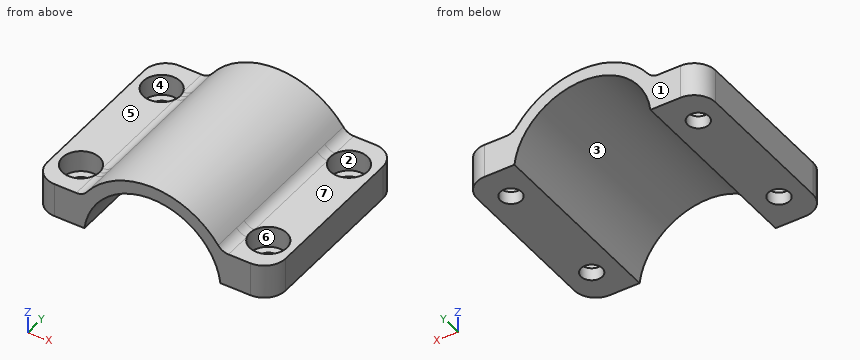
```python
from build123d import *

# Parameters (mm, degrees)
F1_DEPTH = 45
F2_R     = 2.5
F2_R_2   = 4.35
F3_DEPTH = 5
F4_DEPTH = 8.001
F5_R     = 3
F6_R     = 5


with BuildPart() as f1:
    # F0 (on Front) → F1 (new body)
    with BuildSketch(Plane.XZ):
        with BuildLine():
            Line((-28, 10), (-28, 2))
            Line((-28, 2), (-15.975293, 2))
            ThreePointArc((-15.975293, 2), (0, 16.1), (15.975293, 2))
            Line((15.975293, 2), (28, 2))
            Line((28, 2), (28, 10))
            Line((28, 10), (16.272984, 10))
            ThreePointArc((16.272984, 10), (0, 19.1), (-16.272984, 10))
            Line((-16.272984, 10), (-28, 10))
        make_face()
    extrude(amount=F1_DEPTH)

    # F2 (on face) → F3 (cut)
    with BuildSketch(Plane.XY.offset(10)):
        with Locations((-22, -8)):
            Circle(F2_R)
        with Locations((-22, -8)):
            Circle(F2_R_2)
        with Locations((-22, -8)):
            Circle(F2_R, mode=Mode.SUBTRACT)
        with Locations((22, -8)):
            Circle(F2_R)
        with Locations((22, -8)):
            Circle(F2_R_2)
        with Locations((22, -8)):
            Circle(F2_R, mode=Mode.SUBTRACT)
        with Locations((22, -37)):
            Circle(F2_R)
        with Locations((22, -37)):
            Circle(F2_R_2)
        with Locations((22, -37)):
            Circle(F2_R, mode=Mode.SUBTRACT)
        with Locations((-22, -37)):
            Circle(F2_R)
        with Locations((-22, -37)):
            Circle(F2_R_2)
        with Locations((-22, -37)):
            Circle(F2_R, mode=Mode.SUBTRACT)
    extrude(amount=-F3_DEPTH, mode=Mode.SUBTRACT)

    # F2 (on face) → F4 (cut, through all)
    with BuildSketch(Plane.XY.offset(10)):
        with Locations((-22, -8)):
            Circle(F2_R)
        with Locations((22, -8)):
            Circle(F2_R)
        with Locations((-22, -37)):
            Circle(F2_R)
        with Locations((22, -37)):
            Circle(F2_R)
    extrude(amount=-F4_DEPTH, mode=Mode.SUBTRACT)

    # F5
    f5_edges = [f1.edges().sort_by_distance(p)[0] for p in [
        (-16.272984, -22.5, 10),
        (16.272984, -22.5, 10),
    ]]
    fillet(f5_edges, radius=F5_R)

    # F6
    f6_edges = [f1.edges().sort_by_distance(p)[0] for p in [
        (28, -45, 6),
        (28, 0, 6),
        (-28, -45, 6),
        (-28, 0, 6),
    ]]
    fillet(f6_edges, radius=F6_R)


solid = f1.part
```
Geometry: final body of the model. Coordinates: model frame, mm. Face numbers are marked on the shaded views. A direction names the side the tool comes from. Coordinates: 2 decimals unless noted, no trailing zeros. Order: outer loops, then holes, each group sorted by start corner. A loop starts at its lowest first (then second) coordinate and runs counter-clockwise, first axis right, second up. Notation, with made-up numbers: (41.25, 36) -> (61.25, 36) arc R15 cw to (61.25, 50) -> close; hole circle Ø11 at (68, 86.25). An arc over 180 degrees is marked (long way). Write item = value, one per line.
(1) Cut plane A-A on x = -22. Return loops of the section in (y, z).
Solved:
outline = (-45, 2) -> (-39.5, 2) -> (-39.5, 5) -> (-41.35, 5) -> (-41.35, 10) -> (-45, 10) -> close; (-34.5, 2) -> (-10.5, 2) -> (-10.5, 5) -> (-12.35, 5) -> (-12.35, 10) -> (-32.65, 10) -> (-32.65, 5) -> (-34.5, 5) -> close; (-5.5, 2) -> (0, 2) -> (0, 10) -> (-3.65, 10) -> (-3.65, 5) -> (-5.5, 5) -> close
(2) Line query: line 1 (Y direction, x = 22, z = 8.6); line 2 (Y direction, x = -22, z = 2.9); line 3 (X direction, y = -33.5, z = 8.5). Output: solid intervals per line, ascending.
Solved:
line_1 = -45 to -41.35, -32.65 to -12.35, -3.65 to 0
line_2 = -45 to -39.5, -34.5 to -10.5, -5.5 to 0
line_3 = -28 to -24.58, -19.42 to -13.67, 13.67 to 19.42, 24.58 to 28
(3) Pull-direction query (Y, two-part tool) for the marked faces 1, 2, 3 and 4; classes: pulls with the +Y half, pulls with the -Y half, needs draft (parallel to the pull), parting line crosses it, or undercut.
Solved:
face_1 = pulls with the +Y half
face_2 = undercut
face_3 = needs draft
face_4 = undercut
(4) Access query for the marked faces 5, 6 and 7. Directions: +Z, -Z, +X, -X, +Y, -Y. A direction counts if a zero-diameter tool reaches every point of the face in a straight line with its end or side. Return the directions, or none.
Solved:
face_5 = +Z, -X, +Y, -Y
face_6 = +Z
face_7 = +Z, +X, +Y, -Y
(5) Pin query (flat end, axial travel): pin 1 Ø2.5 at (x, y) = (-21.5, -7.5) entering from +Z; pin 2 Ø4 at (x, y) = (-1, -8) entering from +Z; pin 3 Ø6 at (y, z) = (-39.5, 16.5) entering from +X; pin 4 Ø11 at (x, y) = (-22.5, -31) entering from +Z. Return the tip coordinate at first contact, or that it passes through.
Solved:
pin_1 = through
pin_2 = 19.1
pin_3 = 13.51
pin_4 = 10.13
(6) Cut plane D-D on z = 12.5. Return loops of the section in (x, y).
Solved:
outline = (-14.44, -45) -> (-10.15, -45) -> (-10.15, 0) -> (-14.44, 0) -> close; (10.15, -45) -> (14.44, -45) -> (14.44, 0) -> (10.15, 0) -> close
(7) Cut plane B-B on z = 6.25. Return loops of the section in (x, y).
Solved:
outline = (-28, -40) arc R5 ccw to (-23, -45) -> (-14.84, -45) -> (-14.84, 0) -> (-23, 0) arc R5 ccw to (-28, -5) -> close; (14.84, -45) -> (23, -45) arc R5 ccw to (28, -40) -> (28, -5) arc R5 ccw to (23, 0) -> (14.84, 0) -> close; hole circle Ø8.7 at (-22, -37); hole circle Ø8.7 at (-22, -8); hole circle Ø8.7 at (22, -37); hole circle Ø8.7 at (22, -8)
(8) Cut plane C-C on y = -28. Return loops of the section in (x, z), plus the area to 3 significant figures.
Solved:
outline = (-28, 2) -> (-15.98, 2) arc R16.1 cw to (15.98, 2) -> (28, 2) -> (28, 10) -> (17.87, 10) arc R3 cw to (15.45, 11.24) arc R19.1 ccw to (-15.45, 11.24) arc R3 cw to (-17.87, 10) -> (-28, 10) -> close
area = 315 mm²
